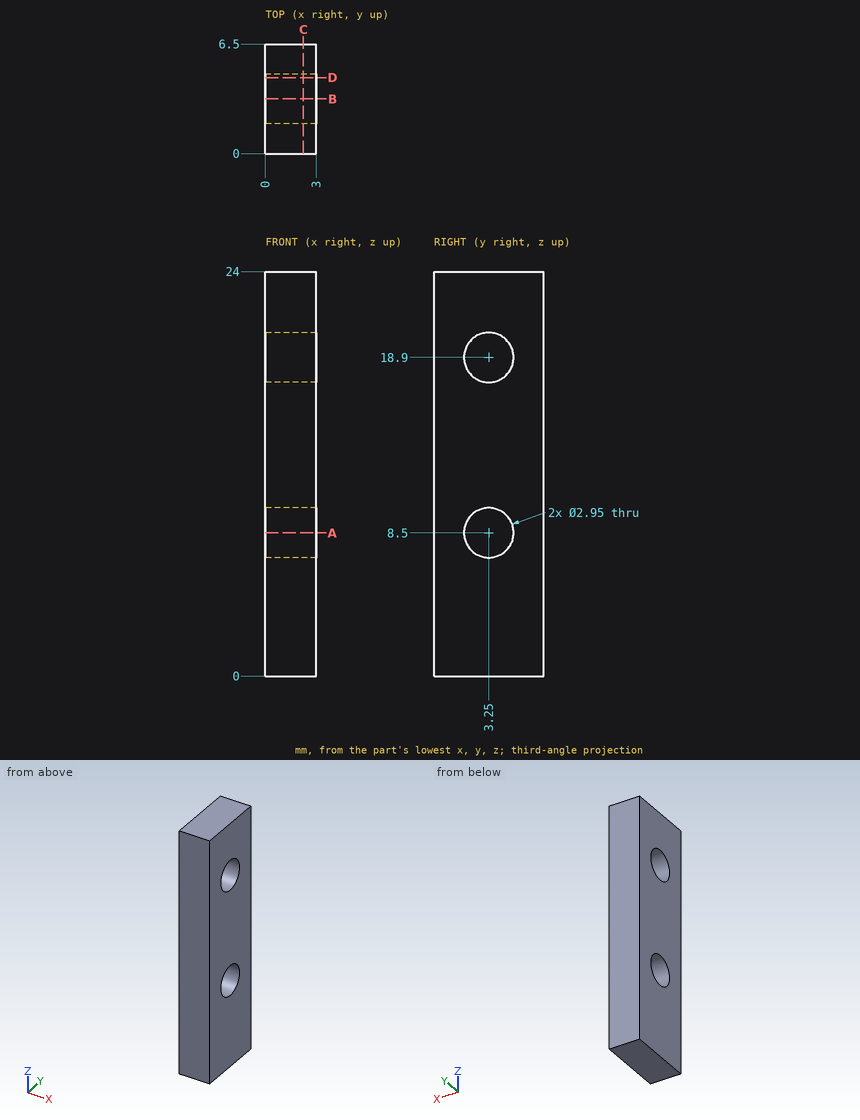
Drawing for the job (mm, zero at the part's lowest x, y, z). Round coordinates to 2 decimals unless told otherwise and drop trailing zeros. Write each loop counter-clockwise with the first axis right and the second up, starting at its lowest first coordinate (ties: lowest second). Pieces come first, ordered by that corner, then holes. Notation, with made-up numbers: (3.5, 56) - (51.5, 56) arc R19 ccw to (51.5, 87) - close; hole circle Ø2 at (38.5, 2.25). An arc over 180 degrees is marked (long way). Write item = value, one per line. Start each with the question number.
Q1. Drop a flat-ended pin along its axis: pin 1 (1.8 mm diameter, centred on y = 3.25, z = 8.5, fed in from +X). Give the stop position or say it passes through.
Q2. Band-saw the part on A-A (z = 8.5). Give the cut face in (x, y) (3 decimals).
Q3. Band-saw the part on B-B (y = 3.25). Give the cut face in (x, z) (3 decimals).
Q4. Probe L1, parallel to Z at x = 1.35, y = 3.25 (3 decimals). List the from-to ranges inside material, lowest first. Write a range as from..to.
Q5. Band-saw the part on D-D (y = 4.5). Give the cut face in (x, z).
Q6. Band-saw the part on C-C (x = 2.25). Give the cut face in (y, z) (3 decimals), then the cut area to 3 significant figures.
Answers below:
q1.pin_1 = through
q2.outline = (0, 0) - (3, 0) - (3, 1.775) - (0, 1.775) - close; (0, 4.725) - (3, 4.725) - (3, 6.5) - (0, 6.5) - close
q3.outline = (0, 0) - (3, 0) - (3, 7.025) - (0, 7.025) - close; (0, 9.975) - (3, 9.975) - (3, 17.425) - (0, 17.425) - close; (0, 20.375) - (3, 20.375) - (3, 24) - (0, 24) - close
q4.L1 = 0..7.025, 9.975..17.425, 20.375..24
q5.outline = (0, 0) - (3, 0) - (3, 7.72) - (0, 7.72) - close; (0, 9.28) - (3, 9.28) - (3, 18.12) - (0, 18.12) - close; (0, 19.68) - (3, 19.68) - (3, 24) - (0, 24) - close
q6.outline = (0, 0) - (6.5, 0) - (6.5, 24) - (0, 24) - close; hole circle Ø2.95 at (3.25, 8.5); hole circle Ø2.95 at (3.25, 18.9)
q6.area = 142 mm2
